from build123d import *

# Parameters (mm, degrees)
SKETCH1_R           = 6.5
BOSS_EXTRUDE1_DEPTH = 13
SKETCH2_R           = 3.225
BOSS_EXTRUDE2_DEPTH = 6.9
SKETCH3_R           = 1.6
BOSS_EXTRUDE3_DEPTH = 14.88
BOSS_EXTRUDE4_DEPTH = 1
CUT_EXTRUDE1_START  = -1
CUT_EXTRUDE1_DEPTH  = 1


with BuildPart() as part:
    # Sketch1 → Boss-Extrude1 (new body)
    with BuildSketch(Plane(origin=(0, 0, 0), x_dir=(1, 0, 0), z_dir=(0, 1, 0))):
        with Locations(Location((0, 0, 0), (0, 0, 90))):
            Circle(SKETCH1_R)
    extrude(amount=BOSS_EXTRUDE1_DEPTH)

    # Sketch2 → Boss-Extrude2 (add)
    with BuildSketch(Plane(origin=(0, 13, 0), x_dir=(1, 0, 0), z_dir=(0, 1, 0))):
        with Locations(Location((0, 0, 0), (0, 0, 90))):
            Circle(SKETCH2_R)
    extrude(amount=BOSS_EXTRUDE2_DEPTH)

    # Sketch3 → Boss-Extrude3 (add)
    with BuildSketch(Plane(origin=(0, 19.9, 0), x_dir=(1, 0, 0), z_dir=(0, 1, 0))):
        with Locations(Location((0, 0, 0), (0, 0, 270))):
            Circle(SKETCH3_R)
    extrude(amount=BOSS_EXTRUDE3_DEPTH)

    # Sketch4 → Boss-Extrude4 (add)
    with BuildSketch(Plane(origin=(0, 13, 0), x_dir=(1, 0, 0), z_dir=(0, 1, 0))):
        with BuildLine():
            ThreePointArc((-1, 5.408326913), (-0.502096593, 5.477033779), (0, 5.5))
            ThreePointArc((0, 5.5), (0.502096593, 5.477033779), (1, 5.408326913))
            Line((1, 5.408326913), (1, 5.5))
            Line((1, 5.5), (1, 6.422616289))
            ThreePointArc((1, 6.422616289), (0, 6.5), (-1, 6.422616289))
            Line((-1, 6.422616289), (-1, 5.5))
            Line((-1, 5.5), (-1, 5.408326913))
        make_face()
        with BuildLine():
            ThreePointArc((1, -5.408326913), (0.502096593, -5.477033779), (0, -5.5))
            ThreePointArc((0, -5.5), (-0.502096593, -5.477033779), (-1, -5.408326913))
            Line((-1, -5.408326913), (-1, -5.5))
            Line((-1, -5.5), (-1, -6.422616289))
            ThreePointArc((-1, -6.422616289), (0, -6.5), (1, -6.422616289))
            Line((1, -6.422616289), (1, -5.5))
            Line((1, -5.5), (1, -5.408326913))
        make_face()
    extrude(amount=BOSS_EXTRUDE4_DEPTH)

    # Sketch5 → Cut-Extrude1 (cut)
    with BuildSketch(Plane(origin=(0, 34.78, 0), x_dir=(1, 0, 0), z_dir=(0, 1, 0)).offset(CUT_EXTRUDE1_START)):
        with BuildLine():
            Line((-1.6, 0), (1.6, 0))
            ThreePointArc((1.6, 0), (1.59507945, 0.125385604), (1.580348063, 0.25))
            Line((1.580348063, 0.25), (-1.580348063, 0.25))
            ThreePointArc((-1.580348063, 0.25), (-1.59507945, 0.125385604), (-1.6, 0))
        make_face()
        with BuildLine():
            ThreePointArc((1.580348063, -0.25), (1.59507945, -0.125385604), (1.6, 0))
            Line((1.6, 0), (-1.6, 0))
            ThreePointArc((-1.6, 0), (-1.59507945, -0.125385604), (-1.580348063, -0.25))
            Line((-1.580348063, -0.25), (1.580348063, -0.25))
        make_face()
    extrude(amount=CUT_EXTRUDE1_DEPTH, mode=Mode.SUBTRACT)


solid = part.part
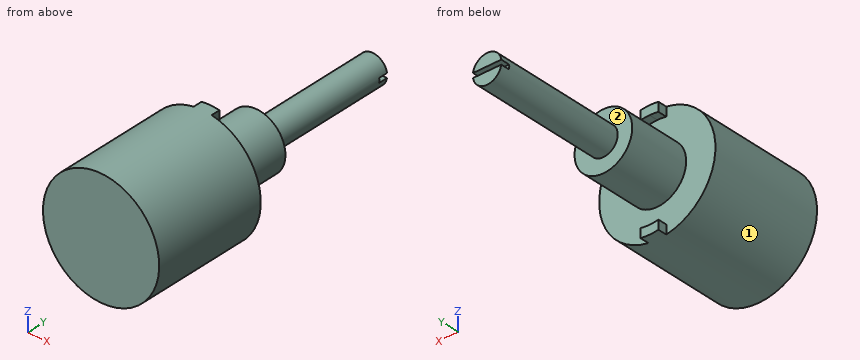
Could you check a few things on this model? Use its own coordinates, in mm. Face numbers are marked on the shaded views. A direction names the side the tool comes from. Give positions to 0.01 mm unless a question says otherwise; leave off trailing zeros. Order: outer loops, then holes, each group sorted by start corner. A loop starts at its lowest first (then second) coordinate and runs counter-clockwise, first axis right, second up. Notation, with made-up numbers: M 45,-24.75 L 63,-24.75 A18 ccw 63,-12.75 Z; hole C 49,84 d1. An arc over 180 degrees is marked long. One line per question, with ' | ' between items.
1. I want a section at B-B (y = 31). List the corners of the cut face in (x, z) for me.
Results:
outline: C 0,0 d3.2
2. I'm going to push flat-ended pins straight in: pin 1 (0.8 mm diameter, centred on x = 0.5, y = 34.5, fed in from -Z); pin 2 (4 mm diameter, centred on y = 13, z = -4, fed in from +X); pin 3 (0.5 mm diameter, centred on y = 13.5, z = 6, fed in from -X). Where does each tip first touch, or does it pass through?
Results:
pin 1: z = -1.6 | pin 2: x = 6.18 | pin 3: x = -1
3. If I drill on line 1 (Y direction, x = 5, z = -2.5); line 2 (Y direction, x = -1.5, z = 2.5); line 3 (X direction, y = 3.5, z = 5.5), over which ranges is the centre line in solid material (lowest first)?
Results:
line 1: 0 to 13 | line 2: 0 to 19.9 | line 3: -3.46 to 3.46
4. For the marked faces 1 and 2, which set-ups out of +Z, -Z, +X, -X, +Y, -Y let a thin tool reach every point of the face, with its end or its side?
Results:
face 1: +Y, -Y | face 2: +Y
5. I want a section at A-A (x = -2). List the corners of the cut face in (y, z) for me, and give its area (3 significant figures).
Results:
outline: M 0,-6.18 L 13,-6.18 L 13,-2.53 L 19.9,-2.53 L 19.9,2.53 L 13,2.53 L 13,6.18 L 0,6.18 Z | area: 196 mm²
6. I want a section at C-C (z = -1). List the corners of the cut face in (x, y) for me.
Results:
outline: M -6.42,0 L 6.42,0 L 6.42,13 L 3.07,13 L 3.07,19.9 L 1.25,19.9 L 1.25,34.78 L -1.25,34.78 L -1.25,19.9 L -3.07,19.9 L -3.07,13 L -6.42,13 Z
7. I want a section at D-D (y = 3). List the corners of the cut face in (x, z) for me, and give its area (3 significant figures).
Results:
outline: C 0,0 d13 | area: 133 mm²
